CAD build for the part. Positions are in the model's coordinates, mm. A direction names the side the tool comes from. Give positions to 0.01 mm unless a question says otherwise; leave off trailing zeros. Loops run counter-clockwise (first coordinate to the right, second up) from the corner with the lowest first, then second, coordinate; pieces in that order, holes last.
Item 1: Which spindle directions (+Z, -Z, +X, -X, +Y, -Y) get a long thin tool onto all of the face, cutting with end or side? Do faces 1 (the cylindrical face through (66.095, -0.608, 0.867)), 2 (the flat face through (1, 0, 0)). Say none if no direction does.
Item 2: Mould opens along Z. For faces 3 (the cylindrical face through (-37.9, 5.09, 18.59)), 4 (the flat face through (1, 5, 19.2)), 5 (the flat face through (1, 5, 18)) say: released by +Z, released by -Z, zero draft, split by the parting line, or undercut.
Item 3: Probe probe 1 along X at (y, z) = (-0.8, 0); probe 2 along Z at (x, y) = (32, 2); probe 3 along Y at (x, z) = (37.5, -16.5). List the from-to ranges inside material, lowest first.
Item 4: Saw through at B-B on z = 0. Give the cut face in (x, y).
Item 5: Saw through at C-C on x = -19. Give the cut face in (y, z).
Item 6: Saw through at A-A on x = -40. Give the cut face in (y, z), plus the area to 3 significant figures.
Item 7: Saw through at D-D on x = 70. Give the cut face in (y, z).
Item 8: Drop flat-ended pins along their axis: P1, Ø1.3, axis at x = -81.5, y = -0.5, coming from the -Z side; P2, Ø1, axis at x = 13, z = -18.5, coming from the +Y side; P3, Ø1, axis at x = 82.5, y = -0.5, coming from the +Z side. Give the stop position or say it passes through.
from build123d import *

# Parameters (mm, degrees)
FLANGE_BASE2_DEPTH      = 90
CORTE_EXTRUS_O3_START   = -90
CORTE_EXTRUS_O3_DEPTH   = 14
CORTE_EXTRUS_O3_START_2 = 76
CORTE_EXTRUS_O3_2_DEPTH = 14
ESBO_O13_R              = 4
CORTE_EXTRUS_O4_DEPTH   = 93.704260959
ESBO_O14_R              = 2.1
CORTE_EXTRUS_O5_DEPTH   = 98.897088823


# Read off the part's stored shape, not the designer's step: Corte-extrusão3
# Sheet-metal steps are written as plain solids
with BuildPart() as part:
    # Esboço1 → Flange-base2 (new, symmetric)
    with BuildSketch(Plane(origin=(0, 0, 0), x_dir=(0, 0, -1), z_dir=(1, 0, 0))):
        with BuildLine():
            Line((-18, 10), (-18, 0.7366))
            ThreePointArc((-18, 0.7366), (-17.784254855, 0.215745145), (-17.2634, 0))
            Line((-17.2634, 0), (17.2634, 0))
            ThreePointArc((17.2634, 0), (17.784254855, 0.215745145), (18, 0.7366))
            Line((18, 0.7366), (18, 3))
            Line((18, 3), (19.2, 3))
            Line((19.2, 3), (19.2, 0.7366))
            ThreePointArc((19.2, 0.7366), (18.632782992, -0.632782992), (17.2634, -1.2))
            Line((17.2634, -1.2), (-17.2634, -1.2))
            ThreePointArc((-17.2634, -1.2), (-18.632782992, -0.632782992), (-19.2, 0.7366))
            Line((-19.2, 0.7366), (-19.2, 10))
            Line((-19.2, 10), (-18, 10))
        make_face()
    extrude(amount=FLANGE_BASE2_DEPTH, both=True)

    # Corte-extrusão3 outline → Corte-extrusão3 (cut)
    with BuildSketch(Plane.YZ.offset(CORTE_EXTRUS_O3_START)):
        with BuildLine():
            Line((-1.2, 17.2634), (0, 17.2634))
            ThreePointArc((0, 17.2634), (0.215745145, 17.784254855), (0.7366, 18))
            Line((0.7366, 18), (10, 18))
            Line((10, 18), (10, 19.2))
            Line((10, 19.2), (0.7366, 19.2))
            ThreePointArc((0.7366, 19.2), (-0.632782992, 18.632782992), (-1.2, 17.2634))
        make_face()
        with BuildLine():
            ThreePointArc((0.7366, -18), (0.215745145, -17.784254855), (0, -17.2634))
            Line((0, -17.2634), (-1.2, -17.2634))
            ThreePointArc((-1.2, -17.2634), (-0.632782992, -18.632782992), (0.7366, -19.2))
            Line((0.7366, -19.2), (3, -19.2))
            Line((3, -19.2), (3, -18))
            Line((3, -18), (0.7366, -18))
        make_face()
    extrude(amount=CORTE_EXTRUS_O3_DEPTH, mode=Mode.SUBTRACT)

    # Corte-extrus_o3 2 outline → Corte-extrus_o3 2 (cut)
    with BuildSketch(Plane.YZ.offset(CORTE_EXTRUS_O3_START_2)):
        with BuildLine():
            Line((-1.2, 17.2634), (0, 17.2634))
            ThreePointArc((0, 17.2634), (0.215745145, 17.784254855), (0.7366, 18))
            Line((0.7366, 18), (10, 18))
            Line((10, 18), (10, 19.2))
            Line((10, 19.2), (0.7366, 19.2))
            ThreePointArc((0.7366, 19.2), (-0.632782992, 18.632782992), (-1.2, 17.2634))
        make_face()
        with BuildLine():
            ThreePointArc((0.7366, -18), (0.215745145, -17.784254855), (0, -17.2634))
            Line((0, -17.2634), (-1.2, -17.2634))
            ThreePointArc((-1.2, -17.2634), (-0.632782992, -18.632782992), (0.7366, -19.2))
            Line((0.7366, -19.2), (3, -19.2))
            Line((3, -19.2), (3, -18))
            Line((3, -18), (0.7366, -18))
        make_face()
    extrude(amount=CORTE_EXTRUS_O3_2_DEPTH, mode=Mode.SUBTRACT)

    # Esboço13 → Corte-extrusão4 (cut, through all)
    with BuildSketch(Plane.XZ.offset(1.2)):
        with Locations(Location((70, 0, 0), (0, 0, 270))):
            Circle(ESBO_O13_R)
    extrude(amount=-CORTE_EXTRUS_O4_DEPTH, mode=Mode.SUBTRACT)

    # Esboço14 → Corte-extrusão5 (cut, through all)
    with BuildSketch(Plane(origin=(0, 0, 18), x_dir=(-1, 0, 0), z_dir=(0, 0, -1))):
        with Locations((-40, 5)):
            Circle(ESBO_O14_R)
        with Locations((40, 5)):
            Circle(ESBO_O14_R)
    extrude(amount=-CORTE_EXTRUS_O5_DEPTH, mode=Mode.SUBTRACT)


solid = part.part
Results below:
1. face 1: +Y, -Y
1. face 2: +X, -X, +Y
2. face 3: zero draft
2. face 4: released by +Z
2. face 5: undercut
3. probe 1: x = -90 to 66, 74 to 90
3. probe 2: z = -19.2 to -18, 18 to 19.2
3. probe 3: y = -1.2 to 0
4. outline: (-90, -1.2) - (66, -1.2) - (66, 0) - (-90, 0) - close; (74, -1.2) - (90, -1.2) - (90, 0) - (74, 0) - close
5. outline: (-1.2, -17.26) arc R1.94 ccw to (0.74, -19.2) - (3, -19.2) - (3, -18) - (0.74, -18) arc R0.74 cw to (0, -17.26) - (0, 17.26) arc R0.74 cw to (0.74, 18) - (10, 18) - (10, 19.2) - (0.74, 19.2) arc R1.94 ccw to (-1.2, 17.26) - close
6. outline: (-1.2, -17.26) arc R1.94 ccw to (0.74, -19.2) - (3, -19.2) - (3, -18) - (0.74, -18) arc R0.74 cw to (0, -17.26) - (0, 17.26) arc R0.74 cw to (0.74, 18) - (2.9, 18) - (2.9, 19.2) - (0.74, 19.2) arc R1.94 ccw to (-1.2, 17.26) - close; (7.1, 18) - (10, 18) - (10, 19.2) - (7.1, 19.2) - close
6. area: 55.3 mm2
7. outline: (-1.2, -17.26) arc R1.94 ccw to (0.74, -19.2) - (3, -19.2) - (3, -18) - (0.74, -18) arc R0.74 cw to (0, -17.26) - (0, -4) - (-1.2, -4) - close; (-1.2, 4) - (0, 4) - (0, 17.26) arc R0.74 cw to (0.74, 18) - (10, 18) - (10, 19.2) - (0.74, 19.2) arc R1.94 ccw to (-1.2, 17.26) - close
8. P1: stops at z = -17.26
8. P2: stops at y = 3
8. P3: stops at z = 17.26
